from build123d import *

# Parameters (mm, degrees)
SKETCH1_W           = 70
SKETCH1_H           = 70
BOSS_EXTRUDE1_DEPTH = 80
CHAMFER1_SIZE       = 10
SKETCH2_W           = 9
SKETCH2_H           = 35
CUT_EXTRUDE1_DEPTH  = 40
SKETCH3_W           = 50
SKETCH3_H           = 80
BOSS_EXTRUDE2_DEPTH = 80


with BuildPart() as part:
    # Sketch1 → Boss-Extrude1 (new body)
    with BuildSketch(Plane(origin=(0, 0, 0), x_dir=(1, 0, 0), z_dir=(0, 1, 0))):
        Rectangle(SKETCH1_W, SKETCH1_H)
    extrude(amount=BOSS_EXTRUDE1_DEPTH)

    # Chamfer1
    chamfer1_edges = [part.edges().sort_by_distance(p)[0] for p in [
        (35, 40, 35),
        (-35, 40, 35),
        (-35, 40, -35),
        (35, 40, -35),
    ]]
    chamfer(chamfer1_edges, length=CHAMFER1_SIZE)

    # Sketch2 → Cut-Extrude1 (cut)
    with BuildSketch(Plane(origin=(0, 0, -35), x_dir=(-1, 0, 0), z_dir=(0, 0, -1))):
        Polygon((-6, 60), (-4.5, 60), (4.5, 60), (6, 60), (6, 70), (-6, 70), align=None)
        with Locations((0, 42.5)):
            Rectangle(SKETCH2_W, SKETCH2_H)
    extrude(amount=-CUT_EXTRUDE1_DEPTH, mode=Mode.SUBTRACT)

    # Sketch3 → Boss-Extrude2 (add)
    with BuildSketch(Plane(origin=(0, 0, -35), x_dir=(-1, 0, 0), z_dir=(0, 0, -1))):
        with Locations((0, 40)):
            Rectangle(SKETCH3_W, SKETCH3_H)
        Polygon((-6, 60), (-6, 70), (6, 70), (6, 60), (4.5, 60), (4.5, 25), (-4.5, 25), (-4.5, 60), align=None, mode=Mode.SUBTRACT)
    extrude(amount=BOSS_EXTRUDE2_DEPTH)


solid = part.part
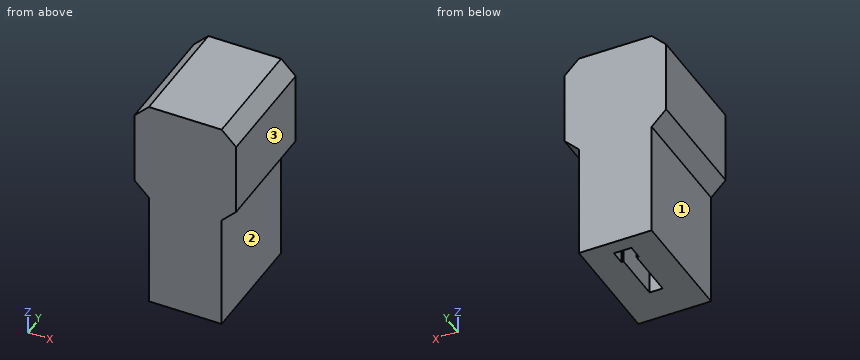
Work out the finished part from the listing and answer in its coordinate system (mm). Face numbers are marked on the shaded views. A direction names the side the tool comes from. Round coordinates to 2 decimals unless told otherwise and drop trailing zeros. Write each loop counter-clockwise with the first axis right and the second up, starting at its lowest first coordinate (ties: lowest second). Pieces come first, ordered by that corner, then holes.
1) A tool of negligible diameter and unlimited length cuts with its end or side. For the marked faces 1, 2 and 3, from which of +Z, -Z, +X, -X, +Y, -Y can it reach the whole face along a straight path? Write none if from no direction.
2) A cutting plane is placed at C-C (z = -53.5). Give the vertices of the cut face in (x, y), plus the area to 4 significant figures.
3) A cutting plane is placed at B-B (x = 1). Give the vertices of the cut face in (y, z).
4) Given pin 1 Ø4 at (y, z) = (33, -59.5) entering from -X; pin 2 Ø11 at (y, z) = (65.5, -33) entering from +X; pin 3 Ø2 at (x, y) = (-0.5, 32.5) entering from -Z, each flat-ended and moving along its own axis, determine where each tip first touches the part or whether it passes through.
5) Straight lines are drawn through the part: line 1 (X direction, y = 28.5, z = -73); line 2 (X direction, y = 68, z = -93); line 3 (Y direction, x = 1, z = -40.5). For each, find the intervals that lie inside material, in ascending order.
6) A cutting plane is placed at A-A (y = 67.5). Give the vertices of the cut face in (x, z).
7) A cutting plane is placed at D-D (z = -4.5). Give the vertices of the cut face in (x, y).
Completed:
1. face 1: -Z, -X, +Y, -Y
1. face 2: -Z, +X, +Y, -Y
1. face 3: +Z, -Z, +X, +Y, -Y
2. outline: (-25, 0) - (25, 0) - (25, 80) - (-25, 80) - close; hole (-6, 60) - (-4.5, 60) - (-4.5, 25) - (4.5, 25) - (4.5, 60) - (6, 60) - (6, 70) - (-6, 70) - close
2. area: 3,565 mm2
3. outline: (0, -115) - (25, -115) - (25, 5) - (70, 5) - (70, -115) - (80, -115) - (80, 35) - (0, 35) - close
4. pin 1: stops at x = -25
4. pin 2: stops at x = 32.5
4. pin 3: stops at z = 5
5. line 1: x = -25 to -4.5, 4.5 to 25
5. line 2: x = -25 to -6, 6 to 25
5. line 3: y = 0 to 25, 70 to 80
6. outline: (-35, -25) - (-25, -35) - (-25, -115) - (-6, -115) - (-6, 5) - (6, 5) - (6, -115) - (25, -115) - (25, -35) - (35, -25) - (35, 25) - (25, 35) - (-25, 35) - (-35, 25) - close
7. outline: (-35, 0) - (35, 0) - (35, 80) - (-35, 80) - close; hole (-6, 60) - (-4.5, 60) - (-4.5, 25) - (4.5, 25) - (4.5, 60) - (6, 60) - (6, 70) - (-6, 70) - close
